Source: CAD feature listing. Evaluate the final solid. Frame: model axes, mm. A direction names the side the tool comes from. Give positions to 0.01 mm unless a question says otherwise; leave off trailing zeros. Order: outer loops, then holes, each group sorted by start corner. A loop starts at its lowest first (then second) coordinate and runs counter-clockwise, first axis right, second up.
```python
from build123d import *

# Parameters (mm, degrees)
BOSS_EXTRUDE1_DEPTH = 9.15
FILLET1_R           = 2.5
SKETCH5_R           = 0.8
CUT_EXTRUDE1_DEPTH  = 15
SKETCH8_R           = 1.25
CUT_EXTRUDE2_DEPTH  = 15
SKETCH9_R           = 5
CUT_EXTRUDE3_DEPTH  = 15
BOSS_EXTRUDE2_START = 10
SKETCH10_R          = 5
SKETCH10_R_2        = 4
BOSS_EXTRUDE2_DEPTH = 10


with BuildPart() as part:
    # Sketch1 → Boss-Extrude1 (new, symmetric)
    with BuildSketch(Plane(origin=(0, 0, 0), x_dir=(1, 0, 0), z_dir=(0, 1, 0))):
        with BuildLine():
            Line((-15, 13.1), (-15, -10.6))
            ThreePointArc((-15, -10.6), (-14.267766953, -12.367766953), (-12.5, -13.1))
            Line((-12.5, -13.1), (12.5, -13.1))
            ThreePointArc((12.5, -13.1), (14.267766953, -12.367766953), (15, -10.6))
            Line((15, -10.6), (15, 13.1))
            ThreePointArc((15, 13.1), (0, 28.1), (-15, 13.1))
        make_face()
    extrude(amount=BOSS_EXTRUDE1_DEPTH, both=True)

    # Fillet1
    # the kernel refuses this fillet: 2.5 mm, written as the material it takes off along each edge
    with BuildSketch(Plane(origin=(-15, 9.15, -28.1), x_dir=(0, -1, 0), z_dir=(0, 0, 1)), Plane(origin=(15, 9.15, 25.6), x_dir=(0, -1, 0), z_dir=(0, 0, -1))) as fillet1_piece_1:
        with BuildLine():
            CenterArc((FILLET1_R, FILLET1_R), FILLET1_R, 180, 90)
            Line((0, FILLET1_R), (-FILLET1_R * 0.02, FILLET1_R))
            Line((-FILLET1_R * 0.02, FILLET1_R), (-FILLET1_R * 0.02, -FILLET1_R * 0.02))
            Line((-FILLET1_R * 0.02, -FILLET1_R * 0.02), (FILLET1_R, -FILLET1_R * 0.02))
            Line((FILLET1_R, -FILLET1_R * 0.02), (FILLET1_R, 0))
        make_face()
    extrude(amount=53.7, mode=Mode.SUBTRACT)

    # Sketch5 → Cut-Extrude1 (cut)
    with BuildSketch(Plane.XZ.offset(9.15)):
        with Locations(Location((0, -23.55, 0), (0, 0, 270))):
            Circle(SKETCH5_R)
        with Locations(Location((-9.04996547, -7.875, 0), (0, 0, 270))):
            Circle(SKETCH5_R)
        with Locations(Location((9.04996547, -7.875, 0), (0, 0, 270))):
            Circle(SKETCH5_R)
    extrude(amount=-CUT_EXTRUDE1_DEPTH, mode=Mode.SUBTRACT)

    # Sketch8 → Cut-Extrude2 (cut)
    with BuildSketch(Plane.XZ.offset(9.15)):
        with Locations(Location((-9.525, -13.1, 0), (0, 0, 270))):
            Circle(SKETCH8_R)
        with Locations(Location((9.525, -13.1, 0), (0, 0, 270))):
            Circle(SKETCH8_R)
    extrude(amount=-CUT_EXTRUDE2_DEPTH, mode=Mode.SUBTRACT)

    # Sketch9 → Cut-Extrude3 (cut)
    with BuildSketch(Plane.XZ.offset(9.15)):
        with Locations(Location((0, -13.1, 0), (0, 0, 270))):
            Circle(SKETCH9_R)
    extrude(amount=-CUT_EXTRUDE3_DEPTH, mode=Mode.SUBTRACT)

    # Sketch10 → Boss-Extrude2 (add)
    with BuildSketch(Plane.XZ.offset(-5.85).offset(BOSS_EXTRUDE2_START)):
        with Locations(Location((0, -13.1, 0), (0, 0, 270))):
            Circle(SKETCH10_R)
        with Locations(Location((0, -13.1, 0), (0, 0, 270))):
            Circle(SKETCH10_R_2, mode=Mode.SUBTRACT)
    extrude(amount=-BOSS_EXTRUDE2_DEPTH)


solid = part.part
```
1) Reachability of faces 1 (the flat face through (0, 0, 13.1)), 2 (the flat face through (4, -4.15, -15)) from +Z, -Z, +X, -X, +Y, -Y: full face, straight path, thin tool, end or side. Return the list, or none.
Report:
face 1: +Z, +X, -X, +Y, -Y
face 2: -Y
2) Draft query along X for faces 3 (the flat face through (9, 5.85, -8)), 4 (the cylindrical face through (14.248, 0.128, 12.387)), 5 (the cylindrical face through (0.33, 0.128, -28.096)), 6 (the flat face through (-0.2, -9.15, -7.8)). Return one class per face: +X half, -X half, draft (parallel to the pull), parting line (faces both ways), or undercut.
Report:
face 3: undercut
face 4: +X half
face 5: parting line
face 6: draft
3) Section query B-B, the plane y = 5. Return the cut outline in (x, z) (3 decimals), and give its area (3 significant figures).
Report:
outline: (-15, -13.1) arc R15 ccw to (15, -13.1) - (15, 10.6) arc R2.5 ccw to (12.5, 13.1) - (-12.5, 13.1) arc R2.5 ccw to (-15, 10.6) - close; hole circle Ø2.5 at (-9.525, -13.1); hole circle Ø1.6 at (-9.05, -7.875); hole circle Ø8 at (0, -13.1); hole circle Ø1.6 at (0, -23.55); hole circle Ø1.6 at (9.05, -7.875); hole circle Ø2.5 at (9.525, -13.1)
area: 1,070 mm2
4) Material intervals for L1, parallel to X at y = -6.95, z = -13.1 (3 decimals); L2, parallel to Z at x = 0.5, y = -7.25; L3, parallel to Z at x = 12.5, y = 8.75, sorted ascending.
Report:
L1: x = -15 to -10.775, -8.275 to -5, 5 to 8.275, 10.775 to 15
L2: z = -28.09 to -24.17, -22.93 to -18.07, -8.13 to 13.1
L3: z = -21.39 to 13.1
5) Section query A-A, the plane x = 0. Return the cut outline in (y, z), and give its area (3 significant figures).
Report:
outline: (-9.15, -28.1) - (9.15, -28.1) - (9.15, 13.1) - (-9.15, 13.1) - (-9.15, -8.1) - (-4.15, -8.1) - (-4.15, -9.1) - (5.85, -9.1) - (5.85, -17.1) - (-4.15, -17.1) - (-4.15, -18.1) - (-9.15, -18.1) - (-9.15, -22.75) - (5.85, -22.75) - (5.85, -24.35) - (-9.15, -24.35) - close
area: 600 mm2
6) Pin query (flat end, axial travel): pin 1 (0.5 mm diameter, centred on x = -9, z = -8, fed in from -Y); pin 2 (6.5 mm diameter, centred on x = -0.5, z = -14.5, fed in from -Y); pin 3 (3 mm diameter, centred on y = 0, z = -18.5, fed in from -X). Return the tip coordinate at first contact, or that it passes through.
Report:
pin 1: stops at y = 5.85
pin 2: stops at y = -4.15
pin 3: stops at x = -14.48
7) Section query C-C, the plane z = -23.55. Return the cut outline in (x, y).
Report:
outline: (-10.76, -9.15) - (-0.8, -9.15) - (-0.8, 5.85) - (0.8, 5.85) - (0.8, -9.15) - (10.76, -9.15) - (10.76, 9.15) - (-10.76, 9.15) - close
8) Section query D-D, the plane y = -5.75. Return the cut outline in (x, z) (3 decimals).
Report:
outline: (-15, -13.1) arc R15 ccw to (15, -13.1) - (15, 10.6) arc R2.5 ccw to (12.5, 13.1) - (-12.5, 13.1) arc R2.5 ccw to (-15, 10.6) - close; hole circle Ø2.5 at (-9.525, -13.1); hole circle Ø1.6 at (-9.05, -7.875); hole circle Ø10 at (0, -13.1); hole circle Ø1.6 at (0, -23.55); hole circle Ø1.6 at (9.05, -7.875); hole circle Ø2.5 at (9.525, -13.1)
